Solid Edge part; units mm, degrees
sketch "Sketch1" plane through (0, 0, 0) normal (0, 0, 1) x (1, 0, 0)
  line L0 (-24.5, 16.25) -> (-24.5, -16.25)
  line L1 (-24.5, -16.25) -> (24.5, -16.25)
  line L2 (24.5, -16.25) -> (24.5, 16.25)
  line L3 (24.5, 16.25) -> (-24.5, 16.25)
extrude "Protrusion1" add sketch "Sketch1" against normal blind 2
sketch "Sketch2" plane through (0, 0, 0) normal (0, 0, 1) x (1, 0, 0)
  line L0 (-23.5, 15.25) -> (-23.5, -15.25)
  line L1 (-23.5, -15.25) -> (23.5, -15.25)
  line L2 (23.5, -15.25) -> (23.5, 15.25)
  line L3 (23.5, 15.25) -> (-23.5, 15.25)
  line L4 (-24.5, 16.25) -> (-24.5, -16.25)
  line L5 (-24.5, -16.25) -> (24.5, -16.25)
  line L6 (24.5, -16.25) -> (24.5, 16.25)
  line L7 (24.5, 16.25) -> (-24.5, 16.25)
extrude "ExtrudedProtrusion_2" add sketch "Sketch2" along normal blind 7.5
sketch "Sketch3" plane through (0, 0, 0) normal (0, 0, 1) x (1, 0, 0)
  line L0 (-17.5, -10) -> (-17.5, 10)
  line L1 (-17.5, 10) -> (-23.5, 10)
  line L2 (-23.5, 10) -> (-23.5, -10)
  line L3 (-23.5, -10) -> (-17.5, -10)
extrude "Cutout1" cut sketch "Sketch3" against normal up to vertex (2 mm away)
sketch "Sketch4" plane through (0, 0, 0) normal (0, 0, 1) x (1, 0, 0)
  circle A0 centre (-20.75, 12.5) radius 0.75
  circle A1 centre (-20.75, -12.5) radius 0.75
  circle A2 centre (20.75, -12.5) radius 0.75
  circle A3 centre (20.75, 12.5) radius 0.75
extrude "Cutout2" cut sketch "Sketch4" against normal up to vertex (2 mm away)
sketch "Sketch5" plane through (0, 0, -2) normal (0, 0, -1) x (1, 0, 0)
  line L0 (-10.05, 5.5) -> (-10.05, -4.5)
  line L1 (-10.05, -4.5) -> (4.7, -4.5)
  line L2 (4.7, -4.5) -> (4.7, 5.5)
  line L3 (4.7, 5.5) -> (-10.05, 5.5)
extrude "ExtrudedCutout_4" cut sketch "Sketch5" against normal blind 1
sketch "Sketch6" plane through (0, 0, -2) normal (0, 0, -1) x (1, 0, 0)
  line L0 (4.7, 5.5) -> (-10.05, 5.5)
  line L1 (-10.05, 5.5) -> (-10.05, -4.5)
  line L2 (-10.05, -4.5) -> (4.7, -4.5)
  line L3 (4.7, -4.5) -> (4.7, 5.5)
extrude "Protrusion2" add sketch "Sketch6" against normal up to vertex (1 mm away)
sketch "Sketch7" plane through (0, 0, -2) normal (0, 0, -1) x (1, 0, 0)
  line L0 (-10.05, -5) -> (4.7, -5)
  line L1 (4.7, -5) -> (4.7, 5)
  line L2 (4.7, 5) -> (-10.05, 5)
  line L3 (-10.05, 5) -> (-10.05, -5)
extrude "ExtrudedCutout_5" cut sketch "Sketch7" against normal blind 1
properties material "Graphite"
Check sheet for the modelled part. Datum: model origin and axes. Units: mm. A direction names the side the tool comes from. Round coordinates to 2 decimals unless told otherwise and drop trailing zeros. Loops run counter-clockwise (first coordinate to the right, second up) from the corner with the lowest first, then second, coordinate; pieces in that order, holes last. Notation, with made-up numbers: M -40,53.5 L -18,53.5 A31 cw -18,77.5 Z; hole C 72,-5 d11. An arc over 180 degrees is marked long. Answer as a JSON object with one key per item and string values.
1. Access from +Z, -Z, +X, -X, +Y, -Y to the whole of each face (thin tool, end or side, straight path). Record for faces 5 (the flat face through (-20, 10, -1)), 6 (the flat face through (-24.5, 0, 3)), 7 (the flat face through (-23.5, 0, 3)), 8 (the flat face through (-2.6, -5, -1.5)).
Reply:
{"face 5": "+Z, -Z", "face 6": "+Z, -Z, -X, +Y, -Y", "face 7": "+Z", "face 8": "-Z"}
2. Mould release check, pull along Y, two halves, no side actions. Record for faces 1 (the flat face through (5, 0, -2)), 2 (the flat face through (0, 15.25, 4)), 3 (the flat face through (0, 16.25, 3)), 4 (the flat face through (0, -16.25, 3)): pulls with the +Y half, pulls with the -Y half, needs draft (parallel to the pull), parting line crosses it, or undercut.
Reply:
{"face 1": "needs draft", "face 2": "undercut", "face 3": "pulls with the +Y half", "face 4": "pulls with the -Y half"}
3. Section check A-A (y = -8.5). Record the boundary of the cut face in (x, z).
Reply:
{"outline": "M -24.5,-2 L -23.5,-2 L -23.5,7.5 L -24.5,7.5 Z; M -17.5,-2 L 24.5,-2 L 24.5,7.5 L 23.5,7.5 L 23.5,0 L -17.5,0 Z"}
4. Scan lines: line 1 (Y direction, x = -20.75, z = -0.6); line 2 (Y direction, x = 20.75, z = -0.45); line 3 (X direction, y = 3, z = 5). Record each from-to range of solid material in increasing order.
Reply:
{"line 1": "y = -16.25 to -13.25, -11.75 to -10, 10 to 11.75, 13.25 to 16.25", "line 2": "y = -16.25 to -13.25, -11.75 to 11.75, 13.25 to 16.25", "line 3": "x = -24.5 to -23.5, 23.5 to 24.5"}
5. Section check D-D (y = -12.5). Record the boundary of the cut face in (x, z), plus the area to 3 significant figures.
Reply:
{"outline": "M -24.5,-2 L -21.5,-2 L -21.5,0 L -23.5,0 L -23.5,7.5 L -24.5,7.5 Z; M -20,-2 L 20,-2 L 20,0 L -20,0 Z; M 21.5,-2 L 24.5,-2 L 24.5,7.5 L 23.5,7.5 L 23.5,0 L 21.5,0 Z", "area": "107 mm²"}
6. Section check B-B (x = 20.75). Record the boundary of the cut face in (y, z), plus the area to 3 significant figures.
Reply:
{"outline": "M -16.25,-2 L -13.25,-2 L -13.25,0 L -15.25,0 L -15.25,7.5 L -16.25,7.5 Z; M -11.75,-2 L 11.75,-2 L 11.75,0 L -11.75,0 Z; M 13.25,-2 L 16.25,-2 L 16.25,7.5 L 15.25,7.5 L 15.25,0 L 13.25,0 Z", "area": "74.0 mm²"}
7. Section check C-C (x = -19.5). Record the boundary of the cut face in (y, z).
Reply:
{"outline": "M -16.25,-2 L -10,-2 L -10,0 L -15.25,0 L -15.25,7.5 L -16.25,7.5 Z; M 10,-2 L 16.25,-2 L 16.25,7.5 L 15.25,7.5 L 15.25,0 L 10,0 Z"}
8. Gauge pin test, flat ends, axial feed: P1, Ø5, axis at x = -9, y = 2.5, coming from the -Z side; P2, Ø12, axis at x = 14.5, y = 9, coming from the +Z side. Record the tip position at first contact, or that the pin passes through.
Reply:
{"P1": "stops at z = -2", "P2": "stops at z = 0"}
